Design review of the part built by this model. Coordinates are the model's own, in mm. Coordinates: 2 decimals unless noted, no trailing zeros. Loops run counter-clockwise (first coordinate to the right, second up) from the corner with the lowest first, then second, coordinate; pieces in that order, holes last.
from build123d import *

# Parameters (mm, degrees)
BOSS_EXTRUDE1_DEPTH = 4.7625
SKETCH2_W           = 84.36568139
SKETCH2_H           = 38.1
CUT_EXTRUDE1_DEPTH  = 4.7625
FILLET1_R           = 5.08


with BuildPart() as part:
    # Sketch1 → Boss-Extrude1 (new body)
    with BuildSketch(Plane(origin=(0, 0, 0), x_dir=(0, 0, -1), z_dir=(1, 0, 0))):
        Polygon((-92.71, 63.5), (-101.6, 63.5), (-127, 0), (-109.22, 0), (-109.22, -4.7625), (-100.33, -4.7625), (-100.33, 0), (-1.27, 0), (-1.27, -4.7625), (7.62, -4.7625), (7.62, 0), (25.4, 0), (0, 63.5), (-8.89, 63.5), (-8.89, 68.2625), (-17.78, 68.2625), (-17.78, 63.5), (-83.82, 63.5), (-83.82, 68.2625), (-92.71, 68.2625), align=None)
    extrude(amount=BOSS_EXTRUDE1_DEPTH)

    # Sketch2 → Cut-Extrude1 (cut)
    with BuildSketch(Plane(origin=(4.7625, 0, 0), x_dir=(0, 0, -1), z_dir=(1, 0, 0))):
        with Locations((-50.818840695, 31.75)):
            Rectangle(SKETCH2_W, SKETCH2_H)
        Polygon((-93.00168139, 12.7), (-93.00168139, 50.8), (-108.24168139, 12.7), align=None)
        Polygon((6.604, 12.7), (-8.636, 50.8), (-8.636, 12.7), align=None)
    extrude(amount=-CUT_EXTRUDE1_DEPTH, mode=Mode.SUBTRACT)

    # Fillet1
    fillet1_edges = [part.edges().sort_by_distance(p)[0] for p in [
        (2.38125, 12.7, 108.24168139),
        (2.38125, 50.8, 93.00168139),
        (2.38125, 50.8, 8.636),
        (2.38125, 12.7, -6.604),
    ]]
    fillet(fillet1_edges, radius=FILLET1_R)


solid = part.part
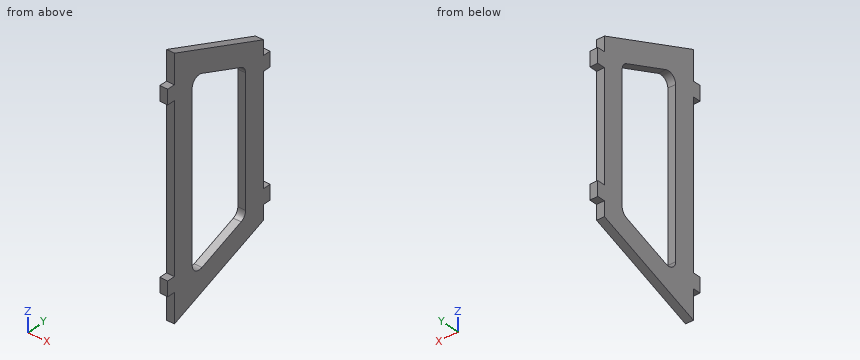
Q1. Take a section at B-B, the plane y = 23.5. Write out the cut boundary in (x, z), then the cut area to 3 significant figures.
Q2. Take a section at D-D, the plane y = 59.5. Write out the cut boundary in (x, z), then the cut area to 3 significant figures.
Q3. Take a section at A-A, the plane z = 43. Write out the cut boundary in (x, y), then the cut area to 3 significant figures.
Q4. For line 1 (Y direction, x = 0.95, z = 15); line 2 (Y direction, x = 2, z = 64.5); line 3 (Z direction, x = 3.7, y = 25.5), list the stretches that pass through material, from the lowest coordinate up.
Q5. Take a section at C-C, the plane x = 3.35. Write out the cut boundary in (y, z), then the cut area to 3 significant figures.
Q6. Clearance check with flat-ended pins moving along their axes: pin 1 Ø2 at (x, y) = (3.5, 55.5) entering from +Z; pin 2 Ø1.4 at (x, y) = (3.5, -3) entering from +Z; pin 3 Ø1.4 at (x, y) = (3, -2) entering from -Z. State where each tip first meets the part, or that it passes through.
Entries:
1. outline: (0, -16) - (4.76, -16) - (4.76, -2.28) - (0, -2.28) - close; (0, 103.92) - (4.76, 103.92) - (4.76, 117.6) - (0, 117.6) - close
1. area: 130 mm2
2. outline: (0, -1.6) - (4.76, -1.6) - (4.76, 103.2) - (0, 103.2) - close
2. area: 499 mm2
3. outline: (0, 0) - (4.76, 0) - (4.76, 12.7) - (0, 12.7) - close; (0, 50.8) - (4.76, 50.8) - (4.76, 63.5) - (0, 63.5) - close
3. area: 121 mm2
4. line 1: y = 0 to 12.7, 50.8 to 68.26
4. line 2: y = 0 to 12.7, 50.8 to 63.5
4. line 3: z = -15.2 to -1.48, 103.12 to 116.8
5. outline: (-4.76, -7.62) - (0, -7.62) - (0, -25.4) - (63.5, 0) - (63.5, 8.89) - (68.26, 8.89) - (68.26, 17.78) - (63.5, 17.78) - (63.5, 83.82) - (68.26, 83.82) - (68.26, 92.71) - (63.5, 92.71) - (63.5, 101.6) - (0, 127) - (0, 109.22) - (-4.76, 109.22) - (-4.76, 100.33) - (0, 100.33) - (0, 1.27) - (-4.76, 1.27) - close; hole (12.7, 0.9) arc R5.08 ccw to (19.67, -3.82) - (47.61, 7.36) arc R5.08 ccw to (50.8, 12.08) - (50.8, 89.56) arc R5.08 ccw to (47.61, 94.28) - (19.67, 105.46) arc R5.08 ccw to (12.7, 100.74) - close
5. area: 4,470 mm2
6. pin 1: stops at z = 105.2
6. pin 2: stops at z = 109.22
6. pin 3: stops at z = -7.62
